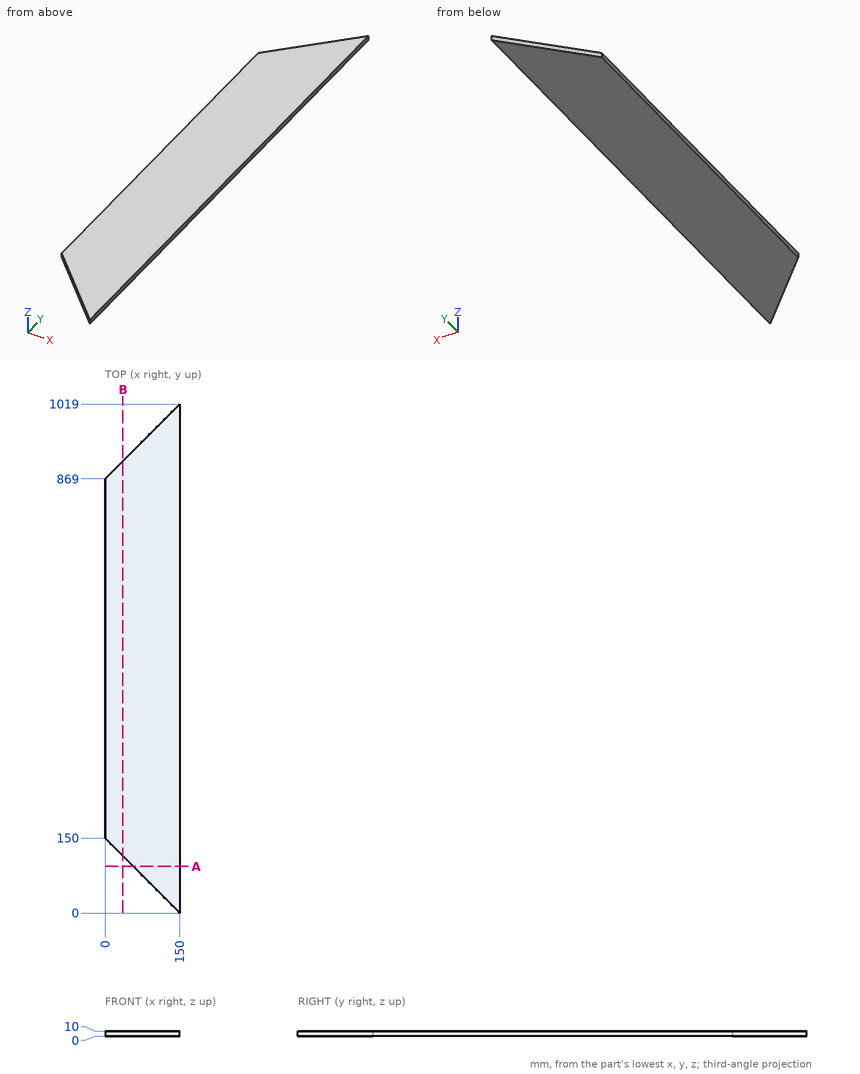
Source: three-view drawing plus pictorial views. Frame: mm from the lowest corner of the part. Coordinates: 2 decimals unless noted, no trailing zeros. Loops run counter-clockwise (first coordinate to the right, second up) from the corner with the lowest first, then second, coordinate; pieces in that order, holes last. Notation, with made-up numbers: (40, -16.5) - (82, -16.5) arc R8 ccw to (82, -11.5) - close; hole circle Ø11 at (-26, -15). An arc over 180 degrees is marked (long way). Answer in a Markdown table with one row per item. Add a question column.
Item 1: Section query B-B on x = 35.5. Return the cut outline in (y, z), then the cut area to 3 significant figures.
Item 2: Line query: line 1 along Y through (x, z) = (17.5, 2.25); line 2 along Y through (x, z) = (135.5, 1.75); line 3 along X through (y, z) = (130.5, 8.5). Output: solid intervals per line, ascending. Write a range as [from, to].
Item 3: Contact query for flat-ended pins moving along their axis: P1, Ø5, axis at x = 61.5, y = 174, coming from the -Z side; P2, Ø2, axis at x = 71.5, z = 8.5, coming from the +Y side; P3, Ø1.5, axis at x = 72.5, z = 8, coming from the -Y side; P4, Ø2, axis at x = 47, z = 5.5, coming from the +Y side. Output: stop coordinate, or through.
Item 4: Section query A-A on y = 93.5. Return the cut outline in (x, z).
Recorded:
| question | item | result |
|---|---|---|
| 1 | outline | (114.5, 0) - (904.5, 0) - (904.5, 10) - (114.5, 10) - close |
| 1 | area | 7,900 mm^2 |
| 2 | line 1 | [132.5, 886.5] |
| 2 | line 2 | [14.5, 1004.5] |
| 2 | line 3 | [19.5, 150] |
| 3 | P1 | z = 0 |
| 3 | P2 | y = 941.5 |
| 3 | P3 | y = 76.75 |
| 3 | P4 | y = 917 |
| 4 | outline | (56.5, 0) - (150, 0) - (150, 10) - (56.5, 10) - close |
